Read the model definition and answer for the solid it produces. Units are mm, in the model's axes. A direction names the side the tool comes from. Give positions to 0.01 mm unless a question says otherwise; leave off trailing zeros. Write each loop counter-clockwise with the first axis right and the second up, starting at its lowest first coordinate (ties: lowest second). Pieces come first, ordered by that corner, then holes. Notation, with made-up numbers: (14, 78) -> (72, 78) arc R29 ccw to (72, 98) -> close; hole circle Ø10 at (56.5, 54.25). An arc over 180 degrees is marked (long way). Put each result on its own line as item: value. Start each with the question number.
from build123d import *

# Parameters (mm, degrees)
SKETCH1_W                      = 10
SKETCH1_H                      = 5
BOSS_EXTRUDE1_DEPTH            = 3
CUT_EXTRUDE9_DEPTH             = 11
SKETCH20_R                     = 1.5
CUT_EXTRUDE11_DEPTH            = 1.2
SKETCH22_R                     = 1.5
SKETCH22_R_2                   = 0.55
CUT_EXTRUDE12_DEPTH            = 0.3
FILLET1_R                      = 0.1
FILLET2_R                      = 0.1
F_1_0MM_DOWEL_HOLE1_AT_2_COUNT = 2
F_1_0MM_DOWEL_HOLE1_AT_2_PITCH = 1.3


with BuildPart() as part:
    # Sketch1 → Boss-Extrude1 (new body)
    with BuildSketch(Plane(origin=(0, 4, 0), x_dir=(-1, 0, 0), z_dir=(0, 1, 0))):
        with Locations((-5, 2.5)):
            Rectangle(SKETCH1_W, SKETCH1_H)
    extrude(amount=-BOSS_EXTRUDE1_DEPTH)

    # Sketch18 → Cut-Extrude9 (cut, through all)
    with BuildSketch(Plane(origin=(10, 0, 0), x_dir=(0, 0, -1), z_dir=(1, 0, 0))):
        Polygon((-3.4, 3.4), (-4, 2.360769515), (-3.4, 2.360769515), (-3.4, 2.110769515), (-1.6, 2.110769515), (-1.6, 2.360769515), (-1, 2.360769515), (-1.6, 3.4), (-1.6, 4), (-3.4, 4), align=None)
    extrude(amount=-CUT_EXTRUDE9_DEPTH, mode=Mode.SUBTRACT)

    # Sketch20 → Cut-Extrude11 (cut)
    with BuildSketch(Plane.ZY):
        with Locations((2.5, 3.060769515)):
            Circle(SKETCH20_R)
    extrude(amount=-CUT_EXTRUDE11_DEPTH, mode=Mode.SUBTRACT)

    # Sketch22 → Cut-Extrude12 (cut)
    with BuildSketch(Plane(origin=(10, 0, 0), x_dir=(0, 0, -1), z_dir=(1, 0, 0))):
        with Locations((-2.5, 3.060769515)):
            Circle(SKETCH22_R)
        with Locations((-2.5, 3.060769515)):
            Circle(SKETCH22_R_2, mode=Mode.SUBTRACT)
    extrude(amount=-CUT_EXTRUDE12_DEPTH, mode=Mode.SUBTRACT)

    # Fillet1
    fillet1_edges = [part.edges().sort_by_distance(p)[0] for p in [
        (5, 1, 5),
        (5, 1, 0),
        (5, 4, 5),
        (5.45, 4, 1.6),
        (5.45, 4, 3.4),
        (5, 4, 0),
        (0.6, 4, 3.669549527),
        (0.6, 4, 1.330450473),
        (9.85, 4, 3.669549527),
        (9.85, 4, 1.330450473),
    ]]
    fillet(fillet1_edges, radius=FILLET1_R)

    # Fillet2
    fillet2_edges = [part.edges().sort_by_distance(p)[0] for p in [
        (10, 3.203038233, 1.006762038),
        (10, 3.203038233, 3.993237962),
        (10, 4, 4.381118968),
        (10, 2.5, 5),
        (10, 1, 2.5),
        (10, 2.5, 0),
        (10, 4, 0.618881032),
        (10, 3.970710678, 4.970710678),
        (10, 3.970710678, 0.029289322),
        (10, 1.029289322, 0.029289322),
        (10, 1.029289322, 4.970710678),
        (10, 3.948758638, 1.22506954),
        (10, 3.948758638, 3.77493046),
        (0, 4, 4.381118968),
        (0, 4, 0.618881032),
        (0, 3.203038233, 1.006762038),
        (0, 2.5, 0),
        (0, 1, 2.5),
        (0, 2.5, 5),
        (0, 3.970710678, 4.970710678),
        (0, 3.970710678, 0.029289322),
        (0, 1.029289322, 0.029289322),
        (0, 1.029289322, 4.970710678),
        (0, 3.948758638, 1.22506954),
        (0, 3.948758638, 3.77493046),
        (0, 3.203038233, 3.993237962),
    ]]
    fillet(fillet2_edges, radius=FILLET2_R)

    # Sketch26 → Ø1.0mm Dowel Hole1 (revolve, cut)
    with BuildSketch(Plane(origin=(0.85, 3.15, 5), x_dir=(0, -1, 0), z_dir=(1, 0, 0))):
        Polygon((0, 0), (0, 0.50043031), (0.5, 0.2), (0.5, 0), align=None)
    f_1_0mm_dowel_hole1 = revolve(axis=Axis((0.85, 3.15, 11.35), (0, 0, -1)), mode=Mode.SUBTRACT)

    # Ø1.0mm Dowel Hole1 at 2: Ø1.0mm Dowel Hole1 ×2
    with Locations(*[(0, -i * F_1_0MM_DOWEL_HOLE1_AT_2_PITCH, 0) for i in range(1, F_1_0MM_DOWEL_HOLE1_AT_2_COUNT)]):
        add(f_1_0mm_dowel_hole1, mode=Mode.SUBTRACT)

    # Sketch28 → UNM0.6 Tapped Hole1 (revolve, cut)
    with BuildSketch(Plane(origin=(0.85, 1, 3.65), x_dir=(0, 0, -1), z_dir=(1, 0, 0))):
        Polygon((0, 0), (0, 2.085193639), (0.225, 1.95), (0.225, 0), align=None)
    unm0_6_tapped_hole1 = revolve(axis=Axis((0.85, -5.35, 3.65), (0, 1, 0)), mode=Mode.SUBTRACT)

    # Mirror1: Ø1.0mm Dowel Hole1, UNM0.6 Tapped Hole1 across plane
    add(f_1_0mm_dowel_hole1.mirror(Plane(origin=(0, 0, 2.5), x_dir=(1, 0, 0), z_dir=(0, 0, -1))), mode=Mode.SUBTRACT)
    add(unm0_6_tapped_hole1.mirror(Plane(origin=(0, 0, 2.5), x_dir=(1, 0, 0), z_dir=(0, 0, -1))), mode=Mode.SUBTRACT)

    # Mirror1 copy 1 sketch → Mirror1 copy 1 (revolve, cut)
    with BuildSketch(Plane(origin=(0.85, 1.85, 0), x_dir=(0, -1, 0), z_dir=(1, 0, 0))):
        Polygon((0, 0), (0, -0.50043031), (0.5, -0.2), (0.5, 0), align=None)
    revolve(axis=Axis((0.85, 1.85, -6.35), (0, 0, -1)), mode=Mode.SUBTRACT)


solid = part.part
1) Straight lines are drawn through the part: line 1 (Y direction, x = 0.85, z = 0.1); line 2 (Z direction, x = 0.85, y = 1.3) (3 decimals); line 3 (X direction, y = 1.45, z = 3.65) (3 decimals). For each, find the intervals that lie inside material, in ascending order. Write a range as [from, to].
2) A cutting plane is placed at B-B on x = 8.25. Give the vertices of the cut face in (y, z).
3) This flat-tipped pin is pushed along its axis until it touches: pin 1 Ø0.5 at (y, z) = (3, 3.5) entering from +X. Where does it stop, or does it pass through?
4) For a pull along X with two mould halves and no side action, classify faces 1 (the face through (5, 4, 4)), 2 (the face through (0.846, 3.237, 4.552)) as pulls with the +X half, pulls with the -X half, needs draft (parallel to the pull), parting line crosses it, or undercut.
5) A cutting plane is placed at A-A on z = 1.35. Give the vertices of the cut face in (x, y) (3 decimals).
6) For faces 3 (the face through (1, 3, 4)), 4 (the face through (6, 2.111, 3)), 5 (the face through (5, 4, 1)), determine the directions among +Z, -Z, +X, -X, +Y, -Y from which every point of the face is accessible in a straight line to the end or side of a thin tool.
Results found:
1. line 1: y = [1, 1.35], [2.35, 2.65], [3.65, 4]
1. line 2: z = [0, 1.125], [1.575, 3.425], [3.875, 5]
1. line 3: x = [0, 0.625], [1.075, 10]
2. outline: (1, 0.1) arc R0.1 ccw to (1.1, 0) -> (3.9, 0) arc R0.1 ccw to (4, 0.1) -> (4, 1.5) arc R0.1 ccw to (3.9, 1.6) -> (3.4, 1.6) -> (2.36, 1) -> (2.36, 1.6) -> (2.11, 1.6) -> (2.11, 3.4) -> (2.36, 3.4) -> (2.36, 4) -> (3.4, 3.4) -> (3.9, 3.4) arc R0.1 ccw to (4, 3.5) -> (4, 4.9) arc R0.1 ccw to (3.9, 5) -> (1.1, 5) arc R0.1 ccw to (1, 4.9) -> close
3. pin 1: stops at x = 9.7
4. face 1: needs draft
4. face 2: undercut
5. outline: (0, 1.1) arc R0.1 ccw to (0.1, 1) -> (0.625, 1) -> (0.625, 2.098) -> (0, 2.098) -> close; (1.075, 1) -> (9.9, 1) arc R0.1 ccw to (10, 1.1) -> (10, 2.098) -> (9.7, 2.098) -> (9.7, 2.361) -> (1.2, 2.361) -> (1.2, 2.098) -> (1.075, 2.098) -> close; (1.2, 2.967) -> (9.7, 2.967) -> (9.7, 4) -> (1.2, 4) -> close
6. face 3: -X
6. face 4: +X, -X, +Y
6. face 5: +Z, -Z, +X, -X, +Y
